from build123d import *

# Parameters (mm, degrees)
SKETCH1_W           = 80
SKETCH1_H           = 20
BOSS_EXTRUDE1_DEPTH = 10
SKETCH2_W           = 80
SKETCH2_H           = 7.5
CUT_EXTRUDE1_DEPTH  = 7.5
BOSS_EXTRUDE2_DEPTH = 10
SKETCH4_W           = 25.799353936
SKETCH4_H           = 15
BOSS_EXTRUDE3_DEPTH = 2.5
CHAMFER1_SIZE       = 7.5


# Some blends are built 0.0001 mm under size
with BuildPart() as part:
    # Sketch1 → Boss-Extrude1 (new, symmetric)
    with BuildSketch(Plane(origin=(0, 0, 0), x_dir=(1, 0, 0), z_dir=(0, 1, 0))):
        Rectangle(SKETCH1_W, SKETCH1_H)
    extrude(amount=BOSS_EXTRUDE1_DEPTH, both=True)

    # Sketch2 → Cut-Extrude1 (cut, symmetric)
    with BuildSketch(Plane(origin=(0, 0, 0), x_dir=(1, 0, 0), z_dir=(0, 1, 0))):
        with Locations((0, 6.25)):
            Rectangle(SKETCH2_W, SKETCH2_H)
        with Locations((0, -6.25)):
            Rectangle(SKETCH2_W, SKETCH2_H)
    extrude(amount=CUT_EXTRUDE1_DEPTH, both=True, mode=Mode.SUBTRACT)

    # Sketch3 → Boss-Extrude2 (add, symmetric)
    with BuildSketch(Plane.XY):
        with BuildLine():
            Line((-40, 10), (-61.684975658, 10))
            Line((-61.684975658, 10), (-61.684975658, -10))
            Line((-61.684975658, -10), (-40, -10))
            ThreePointArc((-40, -10), (-30, 0), (-40, 10))
        make_face()
        Polygon((-46.614378278, 7.5), (-54.114378278, 0), (-46.614378278, -7.5), (-59.184975658, -7.5), (-59.184975658, 7.5), align=None, mode=Mode.SUBTRACT)
    extrude(amount=BOSS_EXTRUDE2_DEPTH, both=True)

    # Sketch4 → Boss-Extrude3 (add, symmetric)
    with BuildSketch(Plane.XY):
        with Locations((-46.28529869, 0)):
            Rectangle(SKETCH4_W, SKETCH4_H)
    extrude(amount=BOSS_EXTRUDE3_DEPTH, both=True)

    # Chamfer1
    # the kernel refuses this chamfer: 7.5 mm, written as the material it adds along each edge
    with BuildSketch(Plane(origin=(-54.114378278, 0, 2.5), x_dir=(0.019442520806014087, 0.019442520806013695, 0.9996219169112968), z_dir=(0.7071067811865405, -0.7071067811865547, 0))) as chamfer1_piece_1_section:
        with BuildLine():
            Line((7.715048964, 0), (-0.424103662, 7.703383451))
            Line((-0.424103662, 7.703383451), (-0.574046949, 7.69925907))
            ThreePointArc((-0.574046949, 7.69925907), (-0.255969203, 3.850483722), (-0.149943288, -0.004124381))
            Line((-0.149943288, -0.004124381), (0.004124381, -0.149943288))
            ThreePointArc((0.004124381, -0.149943288), (3.858732485, -0.043917372), (7.719173345, -0.149943288))
            Line((7.719173345, -0.149943288), (7.715048964, 0))
        make_face()
    chamfer1_piece_1 = extrude(amount=29.894224128, mode=Mode.PRIVATE)
    chamfer1_piece_1 = split(chamfer1_piece_1, bisect_by=Plane(origin=(-52.527454049, -4.471025257, 10), z_dir=(0, 0, -1)), keep=Keep.TOP, mode=Mode.PRIVATE)
    chamfer1_piece_1 = split(chamfer1_piece_1, bisect_by=Plane(origin=(-52.527454049, -7.5, 5.197194263), z_dir=(0, 1, 0)), keep=Keep.TOP, mode=Mode.PRIVATE)
    add(chamfer1_piece_1)
    chamfer1_2_edges = [part.edges().sort_by_distance(p)[0] for p in [
        (-52.899676968, 1.21470131, 2.5),
    ]]
    chamfer(chamfer1_2_edges, length=CHAMFER1_SIZE - 0.0001)  # a hair under: the kernel refuses the full size
    # the kernel refuses this chamfer: 7.5 mm, written as the material it adds along each edge
    with BuildSketch(Plane(origin=(-54.114378278, 0, -2.5), x_dir=(0.019442520806014087, 0.019442520806013695, -0.9996219169112968), z_dir=(0.7071067811865405, -0.7071067811865547, 0))) as chamfer1_3_piece_1_section:
        with BuildLine():
            Line((7.715048964, 0), (-0.424103662, -7.703383451))
            Line((-0.424103662, -7.703383451), (-0.574046949, -7.69925907))
            ThreePointArc((-0.574046949, -7.69925907), (-0.255969203, -3.850483722), (-0.149943288, 0.004124381))
            Line((-0.149943288, 0.004124381), (0.004124381, 0.149943288))
            ThreePointArc((0.004124381, 0.149943288), (3.858732485, 0.043917372), (7.719173345, 0.149943288))
            Line((7.719173345, 0.149943288), (7.715048964, 0))
        make_face()
    chamfer1_3_piece_1 = extrude(amount=29.894224128, mode=Mode.PRIVATE)
    chamfer1_3_piece_1 = split(chamfer1_3_piece_1, bisect_by=Plane(origin=(-52.527454049, -4.471025257, -10), z_dir=(0, 0, 1)), keep=Keep.TOP, mode=Mode.PRIVATE)
    chamfer1_3_piece_1 = split(chamfer1_3_piece_1, bisect_by=Plane(origin=(-52.527454049, -7.5, -5.197194263), z_dir=(0, 1, 0)), keep=Keep.TOP, mode=Mode.PRIVATE)
    add(chamfer1_3_piece_1)
    chamfer1_4_edges = [part.edges().sort_by_distance(p)[0] for p in [
        (-52.899676968, 1.21470131, -2.5),
    ]]
    chamfer(chamfer1_4_edges, length=CHAMFER1_SIZE - 0.0001)  # a hair under: the kernel refuses the full size


solid = part.part
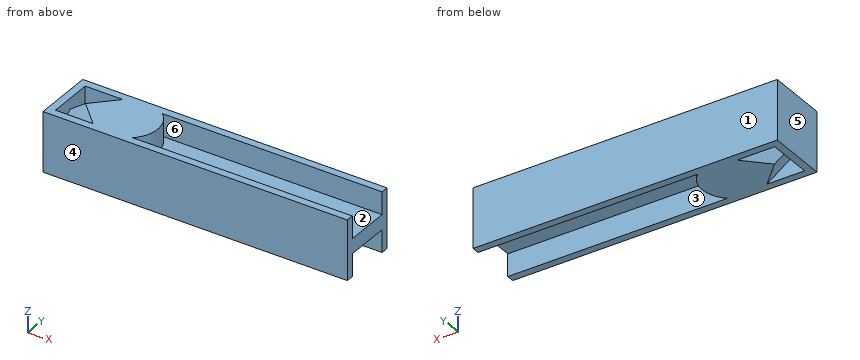
The listing builds one solid part. Answer for the finished solid, in the listing's coordinates (mm). Face numbers are marked on the shaded views. A direction names the side the tool comes from. Give positions to 0.01 mm unless a question says otherwise; leave off trailing zeros. Write each loop counter-clockwise with the first axis right and the second up, starting at its lowest first coordinate (ties: lowest second). Pieces come first, ordered by that corner, then holes. Notation, with made-up numbers: (16.5, -17.5) -> (26.5, -17.5) arc R23 cw to (26.5, 18.5) -> close; hole circle Ø9 at (30, -9). An arc over 180 degrees is marked (long way). Use a Markdown table: item, result.
(1) Section B-B, the plane z = -4.25 is taken. Determine the outline of the cut face in (x, y), then the cut area to 3 significant figures.
Return value:
| item | result |
|---|---|
| outline | (-61.68, -10) -> (40, -10) -> (40, -7.5) -> (-33.39, -7.5) arc R10 ccw to (-33.39, 7.5) -> (40, 7.5) -> (40, 10) -> (-61.68, 10) -> close; hole (-59.18, -7.5) -> (-54.75, -7.5) -> (-59.18, -3.06) -> close; hole (-59.18, 3.06) -> (-54.75, 7.5) -> (-59.18, 7.5) -> close |
| area | 948 mm2 |
(2) Determine the mould class of the marked faces 1, 2, 3 and 4 for opening direction Y: released by +Y, released by -Y, zero draft, split by the parting line, or undercut.
Return value:
| item | result |
|---|---|
| face 1 | released by +Y |
| face 2 | undercut |
| face 3 | undercut |
| face 4 | released by -Y |
(3) Section D-D, the plane z = 4 is taken. Determine the outline of the cut face in (x, y), then the cut area to 3 significant figures.
Return value:
| item | result |
|---|---|
| outline | (-61.68, -10) -> (40, -10) -> (40, -7.5) -> (-33.39, -7.5) arc R10 ccw to (-33.39, 7.5) -> (40, 7.5) -> (40, 10) -> (-61.68, 10) -> close; hole (-59.18, -7.5) -> (-55.1, -7.5) -> (-59.18, -3.41) -> close; hole (-59.18, 3.41) -> (-55.1, 7.5) -> (-59.18, 7.5) -> close |
| area | 951 mm2 |
(4) Find the intervals of material crossed by probe 1 along Y at (x, z) = (7.5, 7.75); probe 2 along X at (y, z) = (2, -7.25); probe 3 along Z at (x, y) = (-15, 3), in increasing order. Write a range as from..to.
Return value:
| item | result |
|---|---|
| probe 1 | -10..-7.5, 7.5..10 |
| probe 2 | -61.68..-59.18, -56..-30.2 |
| probe 3 | -2.5..2.5 |
(5) For the marked faces 5 and 6, determine the directions among +Z, -Z, +X, -X, +Y, -Y from which every point of the face is accessible in a straight line to the end or side of a thin tool.
Return value:
| item | result |
|---|---|
| face 5 | +Z, -Z, -X, +Y, -Y |
| face 6 | +Z, +X |
(6) Section A-A, the plane x = -13 is taken. Determine the outline of the cut face in (y, z), then the cut area to 3 significant figures.
Return value:
| item | result |
|---|---|
| outline | (-10, -10) -> (-7.5, -10) -> (-7.5, -2.5) -> (7.5, -2.5) -> (7.5, -10) -> (10, -10) -> (10, 10) -> (7.5, 10) -> (7.5, 2.5) -> (-7.5, 2.5) -> (-7.5, 10) -> (-10, 10) -> close |
| area | 175 mm2 |
(7) Flat-ended cylindrical pins translate along their axes: P1, Ø4.5, axis at x = -6.5, y = 1.5, coming from the +Z side; P2, Ø6, axis at y = -2.5, z = 7.5, coming from the +X side; P3, Ø1.6, axis at x = -58, y = 6.5, coming from the -Z side. Find the tip coordinate at first contact, or state that the pin passes through.
Return value:
| item | result |
|---|---|
| P1 | z = 2.5 |
| P2 | x = -30 |
| P3 | z = -3.46 |
